The figure shows three views and two pictorial views of one solid part (mm, origin at its lowest corner). Answer the questions. Give positions to 0.01 mm unless a question says otherwise; leave off trailing zeros. Order: outer loops, then holes, each group sorted by start corner. A loop starts at its lowest first (then second) coordinate and runs counter-clockwise, first axis right, second up. Notation, with made-up numbers: (-23.75, 59.5) - (8.25, 59.5) arc R18 ccw to (8.25, 79.5) - close; hole circle Ø11 at (34, -27). An arc over 180 degrees is marked (long way). Answer as CSV lines item,"result". Start each with the question number.
1. Determine the mould class of the marked faces 1 and 2 for opening direction Z: +Z half, -Z half, draft (parallel to the pull), parting line (faces both ways), or undercut.
2. Section C-C on y = 5.25 is taken. Give the vertices of the cut face in (x, z).
3. Section D-D on z = 22.5 is taken. Give the vertices of the cut face in (x, y), and give its area (3 significant figures).
4. Flat-ended cylindrical pins translate along their axes: pin 1 (0.9 mm diameter, centred on x = 6, y = 11.5, fed in from -Z); pin 2 (3 mm diameter, centred on x = 9.5, z = 42, fed in from -Y); pin 3 (3 mm diameter, centred on x = 2, z = 31, fed in from -Y); pin 4 (3 mm diameter, centred on x = 2, z = 39, fed in from +Y). Find the tip coordinate at first contact, or state that the pin passes through.
5. Consider line 1 along Z through (x, y) = (9.25, 11.25); line 2 along Y through (x, z) = (11.5, 19) (1 decimal); line 3 along X through (y, z) = (2, 20) (1 decimal). Determine where each line is inside the solid, lowest interval first. Write a range as [from, to].
6. Section B-B on y = 7.5 is taken. Give the vertices of the cut face in (x, z), and give its area (3 significant figures).
7. Section A-A on x = 6.75 is taken. Give the vertices of the cut face in (y, z) (1 decimal), and give its area (3 significant figures).
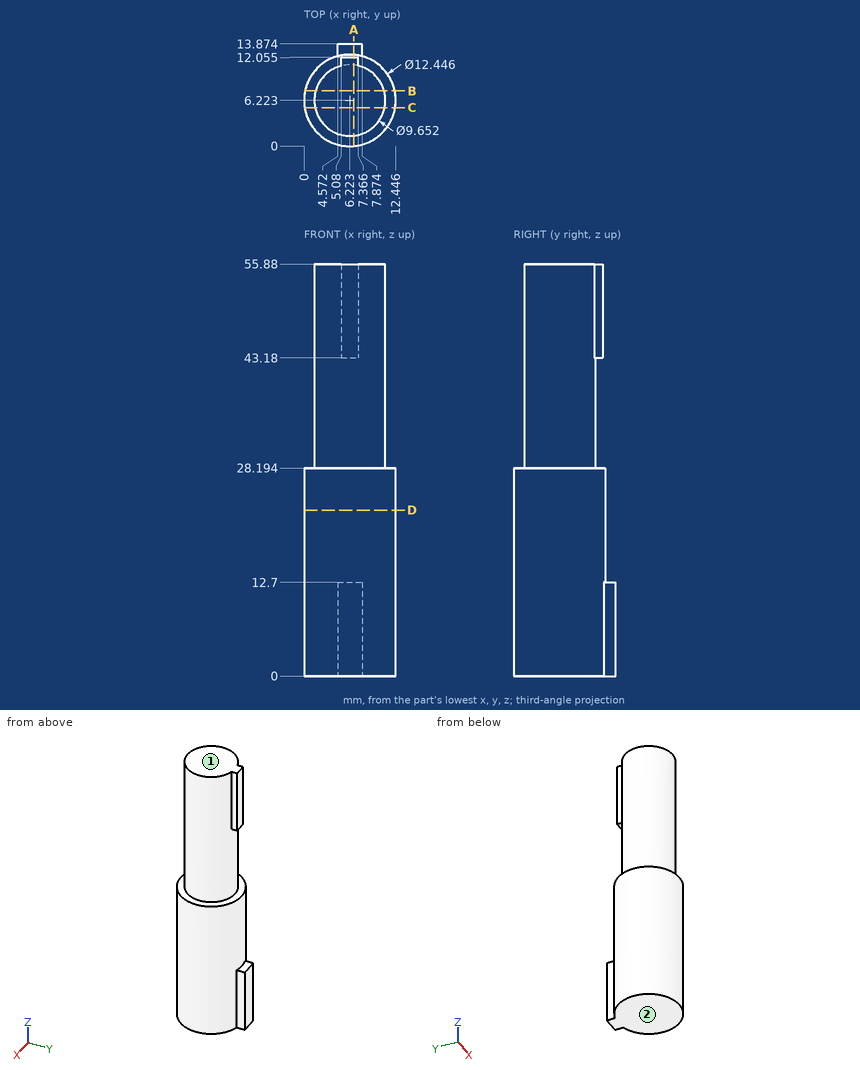
Checks:
1,face 1,"+Z half"
1,face 2,"-Z half"
2,outline,"(0.08, 0) - (12.37, 0) - (12.37, 28.19) - (10.95, 28.19) - (10.95, 55.88) - (1.5, 55.88) - (1.5, 28.19) - (0.08, 28.19) - close"
3,outline,"circle Ø12.45 at (6.22, 6.22)"
3,area,"122 mm²"
4,pin 1,"stops at z = 0"
4,pin 2,"stops at y = 1.74"
4,pin 3,"stops at y = 2.24"
4,pin 4,"stops at y = 10.21"
5,line 1,"z = [0, 28.19]"
5,line 2,"y = [2.9, 9.5]"
5,line 3,"x = [1.7, 10.8]"
6,outline,"(0.13, 0) - (12.31, 0) - (12.31, 28.19) - (10.88, 28.19) - (10.88, 55.88) - (1.57, 55.88) - (1.57, 28.19) - (0.13, 28.19) - close"
6,area,"601 mm²"
7,outline,"(0, 0) - (13.9, 0) - (13.9, 12.7) - (12.4, 12.7) - (12.4, 28.2) - (11, 28.2) - (11, 43.2) - (12.1, 43.2) - (12.1, 55.9) - (1.4, 55.9) - (1.4, 28.2) - (0, 28.2) - close"
7,area,"647 mm²"
